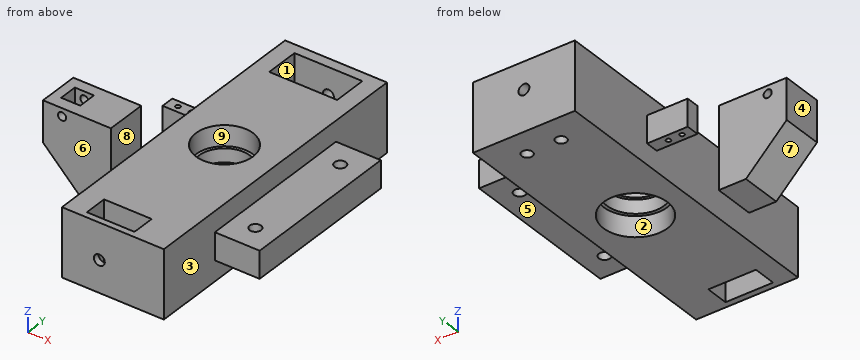
```python
from build123d import *

# Parameters (mm, degrees)
SKETCH1_W                         = 75
SKETCH1_H                         = 50
BE_MAIN_UPRIGHT_BODY_DEPTH        = 221
SKETCH4_R                         = 18.75
CE_THROUGH_HOLE_DEPTH             = 230.667694724
SKETCH2_R                         = 21
CE_INNER_BEARING_DEPTH            = 15
SKETCH3_R                         = 23.5
CE_OUTER_BEARING_DEPTH            = 15
SKETCH7_W                         = 20
SKETCH7_H                         = 120
BE_CALIPER_MOUNT_DEPTH            = 33
SKETCH21_W                        = 30
SKETCH21_H                        = 9.582052631
BE_TEMP_SENSOR_MOUNT_V2_DEPTH     = 10
SKETCH9_W                         = 60
SKETCH9_H                         = 30
BE_TIE_ROD_MOUNT_DEPTH            = 50
SKETCH10_R                        = 4.2
CE_CALIPER_HOLES_DEPTH            = 242.91372429
SKETCH12_R                        = 4
CE_TOP_CLEVIS_HOLES_DEPTH         = 243.893495178
SKETCH33_W                        = 50
SKETCH33_H                        = 25
CE_SIMPLE_TOP_CLEVIS_SPACE_DEPTH  = 30
SKETCH34_R                        = 4
CUT_EXTRUDE12_DEPTH               = 42.5
SKETCH14_W                        = 25
SKETCH14_H                        = 12
CE_BOTTOM_CLEVIS_SPACE_DEPTH      = 243.893495178
SKETCH15_W                        = 25
SKETCH15_H                        = 5
CE_EXPAND_BOTTOM_CLEVIS_DEPTH     = 243.893495178
CE_WIDEN_BOTTOM_CLEVIS_DEPTH      = 240.74121548
CE_WIDEN_BOTTOM_CLEVIS_DEPTH_BACK = 240.74121548
SKETCH16_W                        = 10.007554032
SKETCH16_H                        = 17
CHAMFER1_SIZE                     = 30
SKETCH18_W                        = 14.04398123
SKETCH18_H                        = 13.562779604
CUT_EXTRUDE1_DEPTH                = 20
SKETCH19_R                        = 3
CUT_EXTRUDE2_DEPTH                = 177.032667423
SKETCH22_R                        = 1.7
CUT_EXTRUDE4_DEPTH                = 20
SKETCH31_R                        = 4
CUT_EXTRUDE9_DEPTH                = 31.5
SKETCH35_R                        = 21
CUT_EXTRUDE13_DEPTH               = 10


with BuildPart() as part:
    # Sketch1 → BE - main upright body (new body)
    with BuildSketch(Plane(origin=(0, 0, 0), x_dir=(1, 0, 0), z_dir=(0, 1, 0))):
        Rectangle(SKETCH1_W, SKETCH1_H)
    extrude(amount=BE_MAIN_UPRIGHT_BODY_DEPTH)

    # Sketch4 → CE - Through hole (cut, through all)
    with BuildSketch(Plane.XY.offset(25)):
        with Locations((0, 110.5)):
            Circle(SKETCH4_R)
    extrude(amount=-CE_THROUGH_HOLE_DEPTH, mode=Mode.SUBTRACT)

    # Sketch2 → CE - Inner bearing (cut)
    with BuildSketch(Plane.XY.offset(25)):
        with Locations((0, 110.5)):
            Circle(SKETCH2_R)
    extrude(amount=-CE_INNER_BEARING_DEPTH, mode=Mode.SUBTRACT)

    # Sketch3 → CE - Outer bearing (cut)
    with BuildSketch(Plane(origin=(0, 0, -25), x_dir=(-1, 0, 0), z_dir=(0, 0, -1))):
        with Locations((0, 110.5)):
            Circle(SKETCH3_R)
    extrude(amount=-CE_OUTER_BEARING_DEPTH, mode=Mode.SUBTRACT)

    # Sketch7 → BE - caliper mount (add)
    with BuildSketch(Plane(origin=(37.5, 0, 0), x_dir=(0, 0, -1), z_dir=(1, 0, 0))):
        with Locations((0, 110.5)):
            Rectangle(SKETCH7_W, SKETCH7_H)
    extrude(amount=BE_CALIPER_MOUNT_DEPTH)

    # Sketch21 → BE - temp sensor mount v2 (add, symmetric)
    with BuildSketch(Plane.XY):
        with Locations((-52.5, 144.811784304)):
            Rectangle(SKETCH21_W, SKETCH21_H)
    extrude(amount=BE_TEMP_SENSOR_MOUNT_V2_DEPTH, both=True)

    # Sketch9 → BE - tie rod mount (add)
    with BuildSketch(Plane.ZY.offset(37.5)):
        with Locations((25, 63.5)):
            Rectangle(SKETCH9_W, SKETCH9_H)
    extrude(amount=BE_TIE_ROD_MOUNT_DEPTH)

    # Sketch10 → CE - caliper holes (cut, through all)
    with BuildSketch(Plane.XY.offset(10)):
        with Locations((54, 152.5)):
            Circle(SKETCH10_R)
        with Locations((54, 68.5)):
            Circle(SKETCH10_R)
    extrude(amount=-CE_CALIPER_HOLES_DEPTH, mode=Mode.SUBTRACT)

    # Sketch12 → CE - top clevis holes (cut, through all)
    with BuildSketch(Plane.XY.offset(25)):
        with Locations((-12.5, 201)):
            Circle(SKETCH12_R)
        with Locations((12.5, 201)):
            Circle(SKETCH12_R)
    extrude(amount=-CE_TOP_CLEVIS_HOLES_DEPTH, mode=Mode.SUBTRACT)

    # Sketch33 → CE - simple top clevis space (cut)
    with BuildSketch(Plane.XY.offset(25)):
        with Locations((0, 201)):
            Rectangle(SKETCH33_W, SKETCH33_H)
    extrude(amount=-CE_SIMPLE_TOP_CLEVIS_SPACE_DEPTH, mode=Mode.SUBTRACT)

    # Sketch34 → Cut-Extrude12 (cut)
    with BuildSketch(Plane(origin=(0, 221, 0), x_dir=(1, 0, 0), z_dir=(0, 1, 0))):
        with Locations(Location((0, -5, 0), (0, 0, 90))):
            Circle(SKETCH34_R)
    extrude(amount=-CUT_EXTRUDE12_DEPTH, mode=Mode.SUBTRACT)

    # Sketch14 → CE - bottom clevis space (cut, through all)
    with BuildSketch(Plane.XY.offset(25)):
        with Locations((-9.98, 10.5)):
            Rectangle(SKETCH14_W, SKETCH14_H)
    extrude(amount=-CE_BOTTOM_CLEVIS_SPACE_DEPTH, mode=Mode.SUBTRACT)

    # Sketch15 → CE - expand bottom clevis (cut, through all)
    with BuildSketch(Plane.XY.offset(25)):
        with Locations((-9.98, 19)):
            Rectangle(SKETCH15_W, SKETCH15_H)
    extrude(amount=-CE_EXPAND_BOTTOM_CLEVIS_DEPTH, mode=Mode.SUBTRACT)

    # Sketch16 → CE - widen bottom clevis (cut, two sides: drawn at the far end of the back side and taken through both)
    with BuildSketch(Plane(origin=(2.52, 4.5, 25), x_dir=(1, 0, 0), z_dir=(0, 0, 1)).offset(-CE_WIDEN_BOTTOM_CLEVIS_DEPTH_BACK)):
        with Locations((5.003777016, 8.5)):
            Rectangle(SKETCH16_W, SKETCH16_H)
    extrude(amount=CE_WIDEN_BOTTOM_CLEVIS_DEPTH + CE_WIDEN_BOTTOM_CLEVIS_DEPTH_BACK, mode=Mode.SUBTRACT)

    # Chamfer1
    chamfer1_edges = [part.edges().sort_by_distance(p)[0] for p in [
        (-87.5, 63.5, -5),
    ]]
    chamfer(chamfer1_edges, length=CHAMFER1_SIZE)

    # Sketch18 → Cut-Extrude1 (cut)
    with BuildSketch(Plane.XY.offset(55)):
        with Locations((-73.48, 63.84)):
            Rectangle(SKETCH18_W, SKETCH18_H)
    extrude(amount=-CUT_EXTRUDE1_DEPTH, mode=Mode.SUBTRACT)

    # Sketch19 → Cut-Extrude2 (cut, through all)
    with BuildSketch(Plane(origin=(0, 78.5, 0), x_dir=(1, 0, 0), z_dir=(0, 1, 0))):
        with Locations(Location((-73.48, -49.15, 0), (0, 0, 270))):
            Circle(SKETCH19_R)
    extrude(amount=-CUT_EXTRUDE2_DEPTH, mode=Mode.SUBTRACT)

    # Sketch22 → Cut-Extrude4 (cut)
    with BuildSketch(Plane.XY.offset(10)):
        with Locations((-59.752411208, 144.811784303)):
            Circle(SKETCH22_R)
        with Locations((-49.752411208, 144.811784303)):
            Circle(SKETCH22_R)
    extrude(amount=-CUT_EXTRUDE4_DEPTH, mode=Mode.SUBTRACT)

    # Sketch31 → Cut-Extrude9 (cut)
    with BuildSketch(Plane.XZ):
        with Locations(Location((-9.98, -1.65, 0), (0, 0, 90))):
            Circle(SKETCH31_R)
    extrude(amount=-CUT_EXTRUDE9_DEPTH, mode=Mode.SUBTRACT)

    # Sketch35 → Cut-Extrude13 (cut)
    with BuildSketch(Plane.XY):
        with Locations((0, 110.5)):
            Circle(SKETCH35_R)
    extrude(amount=-CUT_EXTRUDE13_DEPTH, mode=Mode.SUBTRACT)


solid = part.part
```
Could you check a few things on this model? Use its own coordinates, in mm. Face numbers are marked on the shaded views. A direction names the side the tool comes from. Round coordinates to 2 decimals unless told otherwise and drop trailing zeros. Loops run counter-clockwise (first coordinate to the right, second up) from the corner with the lowest first, then second, coordinate; pieces in that order, holes last. Notation, with made-up numbers: M 11.25,77 L 23.25,77 A18 ccw 23.25,90 Z; hole C 71.25,65.25 d8. An arc over 180 degrees is marked long. Write item = value, one per line.
1. Thinking about a two-plate mould opening in X: for the marked faces 1, 2, 3 and 4, which applies, +X half, -X half, draft (parallel to the pull), parting line (faces both ways), or undercut?
Results below:
face_1 = undercut
face_2 = undercut
face_3 = +X half
face_4 = -X half
2. I want a section at A-A, the plane y = 201. Write out the boundary of the cut face in (x, z), and give its area (3 significant figures).
Results below:
outline = M -37.5,-25 L -16.5,-25 L -16.5,-5 L -25,-5 L -25,25 L -37.5,25 Z; M -8.5,-25 L 8.5,-25 L 8.5,-5 L -8.5,-5 Z; M 16.5,-25 L 37.5,-25 L 37.5,25 L 25,25 L 25,-5 L 16.5,-5 Z
area = 1,930 mm²
3. Which directions (+Z, -Z, +X, -X, +Y, -Y) give clear straight access to the entire face, cutting with the end or side of a thin tool? Please do the marked faces 5, 6, 7, 8 and 9.
Results below:
face_5 = -Z, +X, +Y, -Y
face_6 = +Z, -Z, -X, -Y
face_7 = -Z, -X, -Y
face_8 = +Z, +X, +Y, -Y
face_9 = +Z
4. I want a section at B-B, the plane x = -73.48. Write out the boundary of the cut face in (y, z), and give its area (3 significant figures).
Results below:
outline = M 48.5,10.98 L 78.5,10.98 L 78.5,46.15 L 70.62,46.15 L 70.62,35 L 57.06,35 L 57.06,46.15 L 48.5,46.15 Z; M 48.5,52.15 L 57.06,52.15 L 57.06,55 L 48.5,55 Z; M 70.62,52.15 L 78.5,52.15 L 78.5,55 L 70.62,55 Z
area = 951 mm²
5. Will these pins go through, and if not, where does the flat tip stop? P1, Ø5, axis at x = 44, z = -7.5, coming from the +Y side; P2, Ø8.5, axis at y = 13, z = 0, coming from the +X side; P3, Ø7, axis at x = -77, z = 40, coming from the +Y side.
Results below:
P1 = 170.5
P2 = 37.5
P3 = 78.5
6. I need wall thicknesses on probe 1 along X at (y, z) = (152, -5); probe 2 along Y at (x, z) = (-24, 21.5); probe 3 along Y at (x, z) = (0, 7.5). Which ranges of each line are inside material? Lowest first, please.
Results below:
probe_1 = -37.5 to 49.83, 58.17 to 70.5
probe_2 = 0 to 188.5, 213.5 to 221
probe_3 = 0 to 4.5, 21.5 to 91.75, 129.25 to 178.5
7. I want a section at D-D, the plane x = -45.5. Write out the boundary of the cut face in (y, z), and give its area (3 significant figures).
Results below:
outline = M 48.5,-5 L 78.5,-5 L 78.5,55 L 48.5,55 Z; M 140.02,-10 L 149.6,-10 L 149.6,10 L 140.02,10 Z
area = 1,990 mm²
8. I want a section at C-C, the plane y = 152.5. Write out the boundary of the cut face in (x, z), and give its area (3 significant figures).
Results below:
outline = M -37.5,-25 L 37.5,-25 L 37.5,-10 L 49.8,-10 L 49.8,10 L 37.5,10 L 37.5,25 L -37.5,25 Z; M 58.2,-10 L 70.5,-10 L 70.5,10 L 58.2,10 Z
area = 4,240 mm²
